```python
from build123d import *

# Parameters (mm, degrees)
CYLINDER001_R     = 1.5
CYLINDER001_DEPTH = 20
ARRAY_COUNT       = 8
CYLINDER_R        = 11
CYLINDER_DEPTH    = 15
CHAMFER_SIZE      = 1
CHAMFER001_SIZE   = 1
CHAMFER002_SIZE   = 1
CHAMFER003_SIZE   = 1
CHAMFER004_SIZE   = 1
CHAMFER005_SIZE   = 1
CHAMFER006_SIZE   = 1
CHAMFER007_SIZE   = 1


with BuildPart() as array:
    # Cylinder001 → Cylinder001 (new body)
    with BuildSketch(Plane(origin=(11.2, 0, 3), x_dir=(1, 0, 0), z_dir=(0, 0, 1))):
        Circle(CYLINDER001_R)
    extrude(amount=CYLINDER001_DEPTH)

    # Array: Array ×8 about axis
    array_axis = Axis((0, 0, 0), (0, 0, 1))


with BuildPart() as array_1:
    add(array.part)
    for i in range(1, ARRAY_COUNT):
        add(array.part.rotate(array_axis, i * 360 / ARRAY_COUNT))


with BuildPart() as chamfer007:
    # Cylinder → Cylinder (new body)
    with BuildSketch(Plane.XY):
        Circle(CYLINDER_R)
    extrude(amount=CYLINDER_DEPTH)

    # Cut: cut Array
    add(array_1.part, mode=Mode.SUBTRACT)

    # Chamfer
    chamfer_edges = [chamfer007.edges().sort_by_distance(p)[0] for p in [
        (4.209518, -10.162675, 15),
    ]]
    chamfer(chamfer_edges, length=CHAMFER_SIZE)

    # Chamfer001
    chamfer001_edges = [chamfer007.edges().sort_by_distance(p)[0] for p in [
        (10.162675, -4.209518, 15),
    ]]
    chamfer(chamfer001_edges, length=CHAMFER001_SIZE)

    # Chamfer002
    chamfer002_edges = [chamfer007.edges().sort_by_distance(p)[0] for p in [
        (10.162675, 4.209518, 15),
    ]]
    chamfer(chamfer002_edges, length=CHAMFER002_SIZE)

    # Chamfer003
    chamfer003_edges = [chamfer007.edges().sort_by_distance(p)[0] for p in [
        (4.209518, 10.162675, 15),
    ]]
    chamfer(chamfer003_edges, length=CHAMFER003_SIZE)

    # Chamfer004
    chamfer004_edges = [chamfer007.edges().sort_by_distance(p)[0] for p in [
        (-4.209518, 10.162675, 15),
    ]]
    chamfer(chamfer004_edges, length=CHAMFER004_SIZE)

    # Chamfer005
    chamfer005_edges = [chamfer007.edges().sort_by_distance(p)[0] for p in [
        (-10.162675, 4.209518, 15),
    ]]
    chamfer(chamfer005_edges, length=CHAMFER005_SIZE)

    # Chamfer006
    chamfer006_edges = [chamfer007.edges().sort_by_distance(p)[0] for p in [
        (-10.162675, -4.209518, 15),
    ]]
    chamfer(chamfer006_edges, length=CHAMFER006_SIZE)

    # Chamfer007
    chamfer007_edges = [chamfer007.edges().sort_by_distance(p)[0] for p in [
        (-4.209518, -10.162675, 15),
    ]]
    chamfer(chamfer007_edges, length=CHAMFER007_SIZE)


solid = chamfer007.part
```
Design review of the part built by this model. Coordinates are the model's own, in mm. A direction names the side the tool comes from. Give positions to 0.01 mm unless a question says otherwise; leave off trailing zeros. Order: outer loops, then holes, each group sorted by start corner. A loop starts at its lowest first (then second) coordinate and runs counter-clockwise, first axis right, second up. Notation, with made-up numbers: (-31.5, 64) - (8.5, 64) arc R19 ccw to (8.5, 85) - close; hole circle Ø7 at (-28, 61.5). An arc over 180 degrees is marked (long way). Use a Markdown table: item, result. Add a question column.
(1) Add section D-D on z = 1.5. Give the boundary of the cut face in (x, y), then the cut area to 3 significant figures.
(2) Clearance check with flat-ended pins moving along their axes: P1, Ø1, axis at x = -0.5, y = -10, coming from the +Z side; P2, Ø2, axis at y = 8.5, z = 12, coming from the -X side; P3, Ø0.7, axis at x = -7.5, y = 7, coming from the +Z side; P4, Ø1.5, axis at y = -6, z = 10, coming from the +X side. State where each tip first meets the part, or that it passes through.
(3) Mouldability with a two-part tool opening along Y and no side actions: class faces 1 (the face through (0, 0, 15)), 2 (the face through (9.61, 3.93, 14.62)), 3 (the face through (6.88, -6.84, 8.92)) as +Y half, -Y half, draft (parallel to the pull), parting line (faces both ways), or undercut.
(4) Add section A-A on z = 5.5. Give the boundary of the cut face in (x, y), then the cut area to 3 significant figures.
(5) Machinability: for faces 4 (the face through (0, 10, 3)), 5 (the face through (0, -10, 3)), 6 (the face through (-6.88, 6.84, 8.92)), 7 (the face through (-9.7, 0, 8.9)), which of the approach directions +Z, -Z, +X, -X, +Y, -Y give a long, thin tool a straight path to every point of the face, cutting with its end or side? Answer none if there is none.
(6) Wall thickness on probe 1 along X at (y, z) = (8, 11.75); probe 2 along X at (y, z) = (-10, 5.5); probe 3 along Z at (x, y) = (-8, -7.5): over which ranges is each line inside the solid? List them lowest first. Write a range as [from, to].
(7) Add section B-B on x = 0. Give the boundary of the cut face in (y, z).
Report:
| question | item | result |
|---|---|---|
| 1 | outline | circle Ø22 at (0, 0) |
| 1 | area | 380 mm² |
| 2 | P1 | stops at z = 15 |
| 2 | P2 | stops at x = -6.67 |
| 2 | P3 | stops at z = 3 |
| 2 | P4 | stops at x = 9.67 |
| 3 | face 1 | draft |
| 3 | face 2 | +Y half |
| 3 | face 3 | undercut |
| 4 | outline | (-10.9, -1.47) arc R11 ccw to (-8.75, -6.67) arc R1.5 cw to (-6.67, -8.75) arc R11 ccw to (-1.47, -10.9) arc R1.5 cw to (1.47, -10.9) arc R11 ccw to (6.67, -8.75) arc R1.5 cw to (8.75, -6.67) arc R11 ccw to (10.9, -1.47) arc R1.5 cw to (10.9, 1.47) arc R11 ccw to (8.75, 6.67) arc R1.5 cw to (6.67, 8.75) arc R11 ccw to (1.47, 10.9) arc R1.5 cw to (-1.47, 10.9) arc R11 ccw to (-6.67, 8.75) arc R1.5 cw to (-8.75, 6.67) arc R11 ccw to (-10.9, 1.47) arc R1.5 cw to start |
| 4 | area | 357 mm² |
| 5 | face 4 | +Z, +Y |
| 5 | face 5 | +Z, -Y |
| 5 | face 6 | +Z |
| 5 | face 7 | +Z, -X |
| 6 | probe 1 | x = [-6.42, 6.42] |
| 6 | probe 2 | x = [-4.58, -0.9], [0.9, 4.58] |
| 6 | probe 3 | z = [0, 3] |
| 7 | outline | (-11, 0) - (11, 0) - (11, 3) - (9.7, 3) - (9.7, 15) - (-9.7, 15) - (-9.7, 3) - (-11, 3) - close |
